Verification items for the finished model (mm, model axes). A direction names the side the tool comes from. Round coordinates to 2 decimals unless told otherwise and drop trailing zeros. Loops run counter-clockwise (first coordinate to the right, second up) from the corner with the lowest first, then second, coordinate; pieces in that order, holes last. Notation, with made-up numbers: (5, -38.5) - (52, -38.5) arc R14 ccw to (52, -22.5) - close; hole circle Ø11 at (81.25, 5.5). An arc over 180 degrees is marked (long way). Use a Markdown table: item, result. Add a question column.
```python
from build123d import *

# Parameters (mm, degrees)
CROQUIS1_R                   = 10
SALIENTE_EXTRUIR1_DEPTH      = 40
SALIENTE_EXTRUIR1_2_DEPTH    = 40
SALIENTE_EXTRUIR2_DEPTH      = 150
SALIENTE_EXTRUIR2_DEPTH_BACK = 150
CROQUIS2_R                   = 22.5
CROQUIS6_R                   = 22.5
CROQUIS6_R_2                 = 21.5
REVOLUCI_N1_ANGLE            = 90
CORTAR_EXTRUIR2_START        = 60
CROQUIS7_W                   = 34
CROQUIS7_H                   = 26
CORTAR_EXTRUIR2_DEPTH        = 20
CROQUIS8_R                   = 8
SALIENTE_EXTRUIR3_DEPTH      = 40
CORTAR_EXTRUIR3_START        = -27
CROQUIS9_R                   = 7
CORTAR_EXTRUIR3_DEPTH        = 25
CROQUIS4_R                   = 21.5
CORTAR_EXTRUIR1_DEPTH        = 296


with BuildPart() as part:
    # Croquis1 → Saliente-Extruir1 (new body)
    with BuildSketch(Plane(origin=(0, 0, 0), x_dir=(1, 0, 0), z_dir=(0, 1, 0))):
        with Locations(Location((-37.5, 0, 0), (0, 0, 270))):
            Circle(CROQUIS1_R)
    extrude(amount=SALIENTE_EXTRUIR1_DEPTH)



with BuildPart() as body_2:
    # Croquis1 → Saliente-Extruir1 2 (new body)
    with BuildSketch(Plane(origin=(0, 0, 0), x_dir=(1, 0, 0), z_dir=(0, 1, 0))):
        with Locations(Location((37.5, 0, 0), (0, 0, 270))):
            Circle(CROQUIS1_R)
    extrude(amount=SALIENTE_EXTRUIR1_2_DEPTH)


with BuildPart() as part_1:
    add(part.part)

    add(body_2.part)  # Saliente-Extruir2 merges body 2
    # Croquis2 → Saliente-Extruir2 (add, two sides: drawn at the far end of the back side and taken through both)
    with BuildSketch(Plane(origin=(0, 0, 0), x_dir=(0, 0, -1), z_dir=(1, 0, 0)).offset(-SALIENTE_EXTRUIR2_DEPTH_BACK)):
        with Locations((0, 50)):
            Circle(CROQUIS2_R)
    extrude(amount=SALIENTE_EXTRUIR2_DEPTH + SALIENTE_EXTRUIR2_DEPTH_BACK)

    # Croquis6 → Revolución1 (revolve)
    with BuildSketch(Plane(origin=(150, 0, -150), x_dir=(0, 0, 1), z_dir=(-1, 0, 0))):
        with Locations((150, 50.102446163)):
            Circle(CROQUIS6_R)
        with Locations((150, 50.102446163)):
            Circle(CROQUIS6_R_2, mode=Mode.SUBTRACT)
    revoluci_n1 = revolve(axis=Axis((150, 0, 25.625), (0, 0, -1)), revolution_arc=REVOLUCI_N1_ANGLE)

    # Simetría1: Revolución1 across plane
    add(revoluci_n1.mirror(Plane(origin=(0, 0, 0), x_dir=(0, 0, 1), z_dir=(1, 0, 0))))

    # Croquis7 → Cortar-Extruir2 (cut)
    with BuildSketch(Plane(origin=(0, 0, 0), x_dir=(1, 0, 0), z_dir=(0, 1, 0)).offset(CORTAR_EXTRUIR2_START)):
        with Locations((93, 0)):
            Rectangle(CROQUIS7_W, CROQUIS7_H)
    extrude(amount=CORTAR_EXTRUIR2_DEPTH, mode=Mode.SUBTRACT)

    # Croquis8 → Saliente-Extruir3 (add)
    with BuildSketch(Plane.XY):
        with Locations((93, 50)):
            Circle(CROQUIS8_R)
    extrude(amount=-SALIENTE_EXTRUIR3_DEPTH)

    # Croquis9 → Cortar-Extruir3 (cut)
    with BuildSketch(Plane(origin=(0, 0, -40), x_dir=(-1, 0, 0), z_dir=(0, 0, -1)).offset(CORTAR_EXTRUIR3_START)):
        with Locations(Location((-93, 50, 0), (0, 0, 180))):
            Circle(CROQUIS9_R)
    extrude(amount=CORTAR_EXTRUIR3_DEPTH, mode=Mode.SUBTRACT)

    # Croquis4 → Cortar-Extruir1 (cut)
    with BuildSketch(Plane(origin=(150, 0, 0), x_dir=(0, 0, -1), z_dir=(1, 0, 0))):
        with Locations((0, 50)):
            Circle(CROQUIS4_R)
    extrude(amount=-CORTAR_EXTRUIR1_DEPTH, mode=Mode.SUBTRACT)


solid = part_1.part
```
Q1. Go/stop test with flat-tipped pins: pin 1 Ø18 at (y, z) = (62, -2.5) entering from -X; pin 2 Ø23.5 at (y, z) = (37.5, -6) entering from -X; pin 3 Ø18 at (y, z) = (65.5, 3) entering from +X; pin 4 Ø7 at (x, y) = (93.5, 48.5) entering from +Z. Record where each tip stops, or that it passes through.
Q2. Thickness scan on line 1 along X through (y, z) = (50, -34); line 2 along Z through (x, y) = (2, 50); line 3 along X through (y, z) = (43.5, -15). Record the ranges inside material, lowest first.
Q3. Section check B-B on x = 93. Record the cut outline in (y, z).
Q4. Section check C-C on y = 6.5. State how many separate pieces and enclosed holes the cut face has, plus the area to 3 significant figures.
Q5. Set-up check for faces 4 (the face through (-41.33, 14.713, 9.237)), 5 (the face through (91.959, 57.932, -30.382)), 6 (the face through (182, 0, 12)), 7 (the face through (86, 50, -29)): record each of +Z, -Z, +X, -X, +Y, -Y from which the full face is reachable in a straight line by a thin tool's end or side.
Q6. Release check for a two-part mould opening along X. For faces 1 (the face through (4.07, 29.01, 4.66)), 2 (the face through (-146, 50, 0)), 3 (the face through (93, 50, -40)) record: +X half, -X half, draft (parallel to the pull), parting line (faces both ways), or undercut.
Q7. Section check A-A on x = 37.5. Record the cut outline in (y, z).
Determined:
| question | item | result |
|---|---|---|
| 1 | pin 1 | stops at x = -199.49 |
| 1 | pin 2 | stops at x = -217.53 |
| 1 | pin 3 | stops at x = 195.38 |
| 1 | pin 4 | stops at z = 22.5 |
| 2 | line 1 | x = 85 to 86, 100 to 101 |
| 2 | line 2 | z = -22.5 to -21.5, 21.5 to 22.5 |
| 2 | line 3 | x = -200.79 to -198.98, -150 to -146, 198.98 to 200.79 |
| 3 | outline | (42, -40) - (58, -40) - (58, -21.03) arc R22.5 ccw to (68.36, -13) - (67.12, -13) arc R21.5 cw to (57, -20.33) - (57, -38) - (43, -38) - (43, -20.33) arc R21.5 cw (long way) to (67.12, 13) - (68.36, 13) arc R22.5 ccw (long way) to (42, -21.03) - close |
| 4 | separate pieces | 4 |
| 4 | enclosed holes | 2 |
| 4 | area | 908 mm² |
| 5 | face 4 | -Y |
| 5 | face 5 | -Z |
| 5 | face 6 | +Z, -Z, +X, -X, -Y |
| 5 | face 7 | none |
| 6 | face 1 | undercut |
| 6 | face 2 | undercut |
| 6 | face 3 | draft |
| 7 | outline | (0, -10) - (29.84, -10) arc R22.5 ccw (long way) to (29.84, 10) - (0, 10) - close; hole circle Ø43 at (50, 0) |
